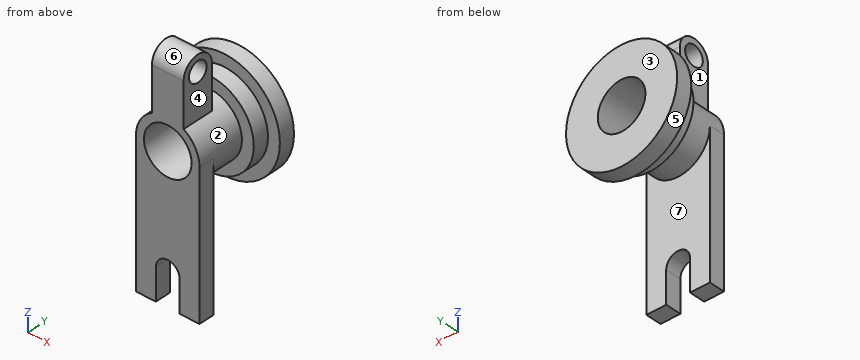
from build123d import *

# Parameters (mm, degrees)
BOSS_EXTRUDE1_DEPTH = 20
SKETCH3_R           = 12.5
BOSS_EXTRUDE2_DEPTH = 20


with BuildPart() as part:
    # Sketch2 → Revolve1 (revolve)
    with BuildSketch(Plane.XY, mode=Mode.PRIVATE) as revolve1_sk:
        Polygon((-30, 0), (-30, 100), (-70, 100), (-70, 80), (-55, 80), (-55, 60), (-40, 60), (-40, 0), align=None)
    revolve(revolve1_sk.sketch.rotate(Axis((0, 0, 0), (0, 1, 0)), 270), axis=Axis((0, 0, 0), (0, 1, 0)))

    # Sketch4 → Boss-Extrude1 (add)
    with BuildSketch(Plane(origin=(0, 0, 0), x_dir=(1, 0, 0), z_dir=(0, 1, 0))):
        with BuildLine():
            Line((-15, 140), (-15, 180))
            Line((-15, 180), (-40, 180))
            Line((-40, 180), (-40, 0))
            ThreePointArc((-40, 0), (0, 40), (40, 0))
            Line((40, 0), (40, 180))
            Line((40, 180), (15, 180))
            Line((15, 180), (15, 140))
            ThreePointArc((15, 140), (0, 125), (-15, 140))
        make_face()
    extrude(amount=BOSS_EXTRUDE1_DEPTH)

    # Sketch3 → Boss-Extrude2 (add, symmetric)
    with BuildSketch(Plane.ZY):
        with BuildLine():
            Line((30, 0), (30, 40))
            Line((30, 40), (90, 40))
            ThreePointArc((90, 40), (110, 20), (90, 0))
            Line((90, 0), (30, 0))
        make_face()
        with Locations((90, 20)):
            Circle(SKETCH3_R, mode=Mode.SUBTRACT)
    extrude(amount=BOSS_EXTRUDE2_DEPTH, both=True)


solid = part.part
Read the model definition and answer for the solid it produces. Units are mm, in the model's axes. Face numbers are marked on the shaded views. A direction names the side the tool comes from. Give positions to 0.01 mm unless a question says otherwise; leave off trailing zeros. Loops run counter-clockwise (first coordinate to the right, second up) from the corner with the lowest first, then second, coordinate; pieces in that order, holes last. Notation, with made-up numbers: (88.25, 20) -> (110.25, 20) arc R25 cw to (110.25, 41) -> close; hole circle Ø8 at (21, 80.25). An arc over 180 degrees is marked (long way). Answer as CSV lines item,"result".
Item 1: Consider line 1 (Z direction, x = 1, y = 22); line 2 (Z direction, x = 1, y = 74.5); line 3 (X direction, y = 62, z = 0). Determine where each line is inside the solid, lowest interval first. Write a range as [from, to].
Returned:
line 1,"z = [-39.99, -29.98], [29.98, 77.66], [102.34, 109.9]"
line 2,"z = [-54.99, -29.98], [29.98, 54.99]"
line 3,"x = [-55, -30], [30, 55]"
Item 2: For the marked faces 1, 2, 3 and 4, determine the directions among +Z, -Z, +X, -X, +Y, -Y from which every point of the face is accessible in a straight line to the end or side of a thin tool.
Returned:
face 1,"+Z, -X, -Y"
face 2,"none"
face 3,"+Z, -Z, +X, -X, +Y"
face 4,"+Z, +X, -Y"
Item 3: Find section A-A on x = 0. Give the vertices of the cut face in (y, z), plus the area to 3 significant figures.
Returned:
outline,"(0, -125) -> (20, -125) -> (20, -40) -> (60, -40) -> (60, -55) -> (80, -55) -> (80, -70) -> (100, -70) -> (100, -30) -> (0, -30) -> close; (0, 30) -> (100, 30) -> (100, 70) -> (80, 70) -> (80, 55) -> (60, 55) -> (60, 40) -> (40, 40) -> (40, 90) arc R20 ccw to (0, 90) -> close; hole circle Ø25 at (20, 90)"
area,"7,640 mm²"
Item 4: Determine the mould class of the marked faces 5, 6 and 7 for opening direction Y: +Y half, -Y half, draft (parallel to the pull), parting line (faces both ways), or undercut.
Returned:
face 5,"draft"
face 6,"parting line"
face 7,"undercut"
Item 5: Find section B-B on y = 28.5. Give the vertices of the cut face in (x, z), plus the area to 3 significant figures.
Returned:
outline,"(-20, 34.64) arc R40 ccw (long way) to (20, 34.64) -> (20, 80.83) -> (-20, 80.83) -> close; (-20, 99.17) -> (20, 99.17) -> (20, 108.1) -> (-20, 108.1) -> close; hole circle Ø60 at (0, 0)"
area,"4,260 mm²"
Item 6: Find section C-C on y = 72.5. Give the vertices of the cut face in (x, z), plus the area to 3 significant figures.
Returned:
outline,"circle Ø110 at (0, 0); hole circle Ø60 at (0, 0)"
area,"6,680 mm²"
Item 7: Find section D-D on z = -75. Give the vertices of the cut face in (x, y), plus the area to 3 significant figures.
Returned:
outline,"(-40, 0) -> (40, 0) -> (40, 20) -> (-40, 20) -> close"
area,"1,600 mm²"
Item 8: Each of these flat-tipped pins is pushed along its axis until it touches: pin 1 (10 mm diameter, centred on y = 5.5, z = -164, fed in from +X); pin 2 (3 mm diameter, centred on x = -17, z = -143.5, fed in from +Y); pin 3 (2 mm diameter, centred on y = 79.5, z = 28, fed in from -X). Where does it stop, or does it pass through?
Returned:
pin 1,"stops at x = 40"
pin 2,"stops at y = 20"
pin 3,"stops at x = -64.53"
